```python
from build123d import *

# Parameters (mm, degrees)
SKETCH1_W           = 12
SKETCH1_H           = 5
BOSS_EXTRUDE1_DEPTH = 5


with BuildPart() as part:
    # Sketch1 → Boss-Extrude1 (new body)
    with BuildSketch(Plane(origin=(0, 0, 0), x_dir=(1, 0, 0), z_dir=(0, 1, 0))):
        with BuildLine():
            Line((-50, 40), (50, 40))
            ThreePointArc((50, 40), (57.071067812, 37.071067812), (60, 30))
            Line((60, 30), (60, -30))
            ThreePointArc((60, -30), (57.071067812, -37.071067812), (50, -40))
            Line((50, -40), (-50, -40))
            ThreePointArc((-50, -40), (-57.071067812, -37.071067812), (-60, -30))
            Line((-60, -30), (-60, 30))
            ThreePointArc((-60, 30), (-57.071067812, 37.071067812), (-50, 40))
        make_face()
        with Locations((-24, 0)):
            Rectangle(SKETCH1_W, SKETCH1_H, mode=Mode.SUBTRACT)
        with Locations((24, 0)):
            Rectangle(SKETCH1_W, SKETCH1_H, mode=Mode.SUBTRACT)
        Rectangle(SKETCH1_W, SKETCH1_H, mode=Mode.SUBTRACT)
    extrude(amount=BOSS_EXTRUDE1_DEPTH)


solid = part.part
```
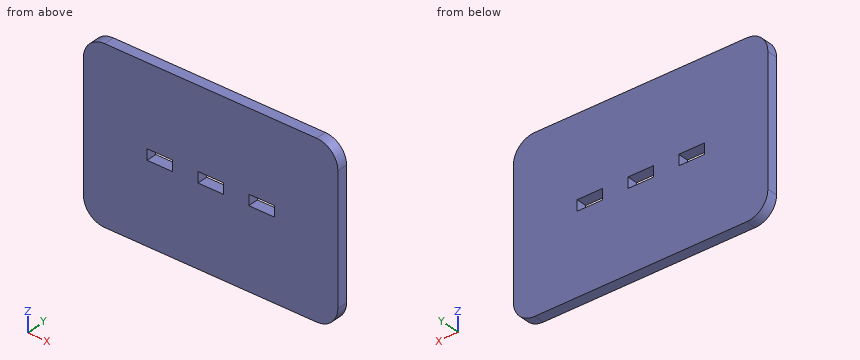
Could you check a few things on this model? Use its own coordinates, in mm. Round coordinates to 2 decimals unless told otherwise and drop trailing zeros. Loops run counter-clockwise (first coordinate to the right, second up) from the corner with the lowest first, then second, coordinate; pieces in that order, holes last. Notation, with made-up numbers: (85, 60) - (119, 60) arc R25 ccw to (119, 76) - close; hole circle Ø8 at (-4.5, 24.5). An arc over 180 degrees is marked (long way). Answer in a Markdown table with one row per item. Add a question column.
(1) If we section it at A-A (x = -23): Please give me the cut outline in (y, z).
(2) If we section it at B-B (y = 1.85): Please give me the cut outline in (x, z), plus the area to 3 significant figures.
(3) I need wall thicknesses on line 1 along Z through (x, y) = (-2, 1.8); line 2 along X through (y, z) = (1.95, -30.5); line 3 along X through (y, z) = (3, -35). Which ranges of each line are inside material? Lowest first, please.
Model answer:
| question | item | result |
|---|---|---|
| 1 | outline | (0, -40) - (5, -40) - (5, -2.5) - (0, -2.5) - close; (0, 2.5) - (5, 2.5) - (5, 40) - (0, 40) - close |
| 2 | outline | (-60, -30) arc R10 ccw to (-50, -40) - (50, -40) arc R10 ccw to (60, -30) - (60, 30) arc R10 ccw to (50, 40) - (-50, 40) arc R10 ccw to (-60, 30) - close; hole (-30, -2.5) - (-18, -2.5) - (-18, 2.5) - (-30, 2.5) - close; hole (-6, -2.5) - (6, -2.5) - (6, 2.5) - (-6, 2.5) - close; hole (18, -2.5) - (30, -2.5) - (30, 2.5) - (18, 2.5) - close |
| 2 | area | 9,330 mm² |
| 3 | line 1 | z = -40 to -2.5, 2.5 to 40 |
| 3 | line 2 | x = -59.99 to 59.99 |
| 3 | line 3 | x = -58.66 to 58.66 |
